Autodesk Inventor part; units mm, degrees
ref_plane "YZ Plane" through (0, 0, 0) normal (1, 0, 0) x (0, 1, 0)
ref_plane "XZ Plane" through (0, 0, 0) normal (0, 1, 0) x (-1, 0, 0)
ref_plane "XY Plane" through (0, 0, 0) normal (0, 0, 1) x (1, 0, 0)
sketch "Skizze2" plane through (0, 0, 0) normal (0, 0, 1) x (1, 0, 0)
  line L0 (-19.9249, 0) -> (3.9249, 0)
  line L1 (0, -18.1036) -> (0, 108.6213)
  circle A0 centre (-8, 65) radius 2.7
  line L2 (0, 0) -> (0, 87.5)
  arc A1 (0, 87.5) -> (-2.5, 90) centre (-2.5, 87.5) ccw
  line L3 (-13.5, 90) -> (-2.5, 90)
  arc A2 (-13.5, 90) -> (-16, 87.5) centre (-13.5, 87.5) ccw
  line L4 (0, 42.5) -> (0, 87.5)
  line L5 (-16, 40) -> (-16, 87.5)
  line L6 (0, 40) -> (-16, 40)
  point P0 (-8, 90)
  dimension "d4" = 2.5
  dimension "d5" = 2.5
  dimension "d6" = 5.4
  dimension "d8" = 25
  dimension "d17" = 2.5
  dimension "d18" = 2.5
  dimension "d19" = 2.5
  dimension "d144" = 25
extrude "Extrusion1" add sketch "Skizze2" along normal mid plane 8
sketch "Skizze7" plane through (0, 0, -4) normal (0, 0, -1) x (-1, 0, 0)
  arc A0 (16, 87.5) -> (13.5, 90) centre (13.5, 87.5) ccw
  line L0 (13.5, 90) -> (2.5, 90)
  arc A1 (2.5, 90) -> (0, 87.5) centre (2.5, 87.5) ccw
  line L1 (0, 87.5) -> (0, 40)
  circle A2 centre (8, 65) radius 2.7
  circle A3 centre (8, 65) radius 6.5
  line L2 (8, 85) -> (8, 45)
  line L3 (13, 82.2483) -> (13, 48.2483)
  line L4 (3, 48.3648) -> (3, 82.3648)
  line L5 (16, 40) -> (16, 87.5)
  line L6 (0, 40) -> (16, 40)
  circle A4 centre (8, 82) radius 3
  circle A5 centre (8, 48) radius 3
  line L7 (-2, 82) -> (18, 82)
  line L8 (-2, 48) -> (18, 48)
  line L9 (5, 48) -> (3, 60.8467)
  line L10 (11, 48) -> (13, 60.8467)
  line L11 (3, 69.1533) -> (5, 82)
  line L12 (13, 69.1533) -> (11, 82)
  point P0 (0, 0)
  point P1 (8, 65)
  dimension "d133" = 13
  dimension "d136" = 20
  dimension "d137" = 20
  dimension "d194" = 6
  dimension "d195" = 6
  dimension "d196" = 3
  dimension "d197" = 3
  dimension "d198" = 10
  dimension "d199" = 20
  dimension "d200" = 20
extrude "Extrusion5" cut sketch "Skizze7" against normal blind 4 contours L8 L2 A5 | A5 L2 L8 | A5 L2 A3 L10 | L3 A3 L2 A2 | A3 L3 | A3 L2 A4 L12 | L7 L2 A4 | A4 L2 L7 | A5 L8 L2 | A5 L9 A3 L2 | L2 L8 A5 | L2 A2 A3 L4 | A3 L11 A4 L2 | L2 L7 A4 | A4 L7 L2 | L4 A3
fillet "Rundung2" radius 2.5 2 edges at (0, 40, 0) (-16, 40, 0)
sketch "Skizze12" plane through (-16, 40, 4) normal (-1, 0, 0) x (0, 0, 1)
  line L0 (0, 47.5) -> (0, 0)
  line L1 (-8, 0) -> (-8, 47.5)
  line L2 (0, 47.5) -> (0, 2.5)
  line L3 (-8, 47.5) -> (0, 47.5)
  line L4 (-8, 2.5) -> (-8, 47.5)
  line L5 (0, 6) -> (-8, 6)
  line L6 (-8, 6) -> (-8, 14)
  line L7 (-8, 14) -> (0, 14)
  line L8 (0, 14) -> (0, 6)
  line L9 (0, 2.5) -> (-8, 2.5)
  point P0 (-4, -40)
  point P1 (0, 8)
  point P2 (-4, 20.6699)
  point P3 (0, 14)
  dimension "d184" = 8
extrude "Extrusion10" add sketch "Skizze12" along normal blind 80 contours L0 L5 L1 L7
sketch "Skizze17" plane through (-16, 54, 4) normal (0, 1, 0) x (1, 0, 0)
  line L0 (-80, 0) -> (-80, 8)
  line L1 (-72, 29) -> (-80, 29)
  line L2 (-72, -21) -> (-80, -21)
  line L3 (-80, 29) -> (-80, -21)
  line L4 (-72, 29) -> (-72, -21)
  line L5 (0, 8) -> (0, 0)
  line L6 (0, 8) -> (-80, 8)
  line L7 (-80, 0) -> (-80, 8)
  line L8 (0, 0) -> (-80, 0)
  line L9 (-80, 4) -> (0, 4)
  point P0 (16, 4)
  point P1 (-80, 8)
  dimension "d187" = 50
  dimension "d188" = 8
extrude "Extrusion15" add sketch "Skizze17" against normal blind 8 contours L8 L4 L2 L3 | L0 L9 L4 L8 | L0 L6 L4 L9 | L3 L1 L4 L6
chamfer "Fasen10" distance 3 angle 45 4 edges at (-16, 46, 0) (-16, 54, 0) (-88, 50, -4) (-88, 50, 4)
sketch "Skizze18" plane through (0, 0, 4) normal (0, 0, 1) x (1, 0, 0)
  circle A0 centre (-8, 65) radius 2.7
  arc A1 (-13, 69.1533) -> (-13, 60.8467) centre (-8, 65) ccw
  line L0 (-11, 82) -> (-13, 69.1533)
  arc A2 (-5, 82) -> (-11, 82) centre (-8, 82) ccw
  line L1 (-3, 69.1533) -> (-5, 82)
  arc A3 (-3, 60.8467) -> (-3, 69.1533) centre (-8, 65) ccw
  line L2 (-5, 48) -> (-3, 60.8467)
  arc A4 (-11, 48) -> (-5, 48) centre (-8, 48) ccw
  line L3 (-13, 60.8467) -> (-11, 48)
  circle A5 centre (-8, 65) radius 2.7
  point P0 (0, 0)
extrude "Extrusion16" cut sketch "Skizze18" against normal blind 0.0001
sketch "Skizze19" plane through (-13.5, 90, 4) normal (0, 1, 0) x (1, 0, 0)
  line L0 (11, 0) -> (0, 0)
  line L1 (0, 8) -> (11, 8)
  line L2 (11, 8) -> (11, 0)
  line L3 (13.5, 0) -> (11, 0)
  line L4 (13.5, 8) -> (13.5, 0)
  line L5 (11, 8) -> (13.5, 8)
  line L6 (-2.5, 8) -> (-2.5, 0)
  line L7 (0, 0) -> (-2.5, 0)
  line L8 (0, 0) -> (0, 8)
  line L9 (-2.5, 8) -> (0, 8)
  point P0 (13.5, 4)
extrude "Extrusion17" cut sketch "Skizze19" against normal blind 8
properties part number "Gripper neu"
Read the model definition and answer for the solid it produces. Units are mm, in the model's axes. A direction names the side the tool comes from. Coordinates: 2 decimals unless noted, no trailing zeros. Write each loop counter-clockwise with the first axis right and the second up, starting at its lowest first coordinate (ties: lowest second). Pieces come first, ordered by that corner, then holes. Notation, with made-up numbers: (85, 74.5) - (112, 74.5) arc R10 cw to (112, 84.5) - close; hole circle Ø9 at (2, 24.5). An arc over 180 degrees is marked (long way). Answer as a JSON object with one key per item and string values. Group by question number.
1. A cutting plane is placed at B-B (z = -2). Determine the outline of the cut face in (x, y).
2. The mould has two halves that part along X. Classify faces 4 (the cylindrical face through (-14.5, 64.9, -2)), 5 (the flat face through (0, 62, 0)), 6 (the flat face through (-33, 53, 4)): +X half, -X half, draft (parallel to the pull), parting line (faces both ways), or undercut.
3. Which of the six approach directions +Z, -Z, +X, -X, +Y, -Y give full straight-line access (tool end or side, diameter ignored) to faces 1 (the cylindrical face through (-1.5, 65.1, -2)), 2 (the flat face through (-88, 50, -16)), 3 (the flat face through (-69, 46, 0))?
4. Each of these flat-tipped pins is pushed along its axis until it touches: P1, Ø8, axis at x = -66, y = 49.5, coming from the +Z side; P2, Ø25, axis at x = -53, z = -2.5, coming from the -Y side; P3, Ø9, axis at y = 51, z = 15, coming from the +X side. Where does it stop, or does it pass through?
5. A cutting plane is placed at D-D (x = -51.5). Determine the outline of the cut face in (y, z).
6. Consider L1, parallel to X at y = 65, z = 1; L2, parallel to Y at x = -8, z = 1; L3, parallel to X at y = 70, z = 3. Determine where each line is inside the solid, lowest interval first. Write a range as [from, to].
Worked out:
{
 "1": {"outline": "(-96, 46) - (-19, 46) - (-16, 43) - (-16, 42.5) arc R2.5 ccw to (-13.5, 40) - (-2.5, 40) arc R2.5 ccw to (0, 42.5) - (0, 82) - (-5, 82) - (-3, 69.15) arc R6.5 cw to (-3, 60.85) - (-5, 48) arc R3 cw to (-11, 48) - (-13, 60.85) arc R6.5 cw to (-13, 69.15) - (-11, 82) - (-16, 82) - (-16, 57) - (-19, 54) - (-96, 54) - close"},
 "2": {"face 4": "undercut", "face 5": "+X half", "face 6": "draft"},
 "3": {"face 1": "-Z", "face 2": "-Z, +X, +Y, -Y", "face 3": "+Z, -Z, -X, -Y"},
 "4": {"P1": "stops at z = 4", "P2": "stops at y = 46", "P3": "stops at x = -88"},
 "5": {"outline": "(46, -4) - (54, -4) - (54, 4) - (46, 4) - close"},
 "6": {"L1": "x = [-16, -10.7], [-5.3, 0]", "L2": "y = [40, 62.3], [67.7, 82]", "L3": "x = [-16, 0]"}
}
